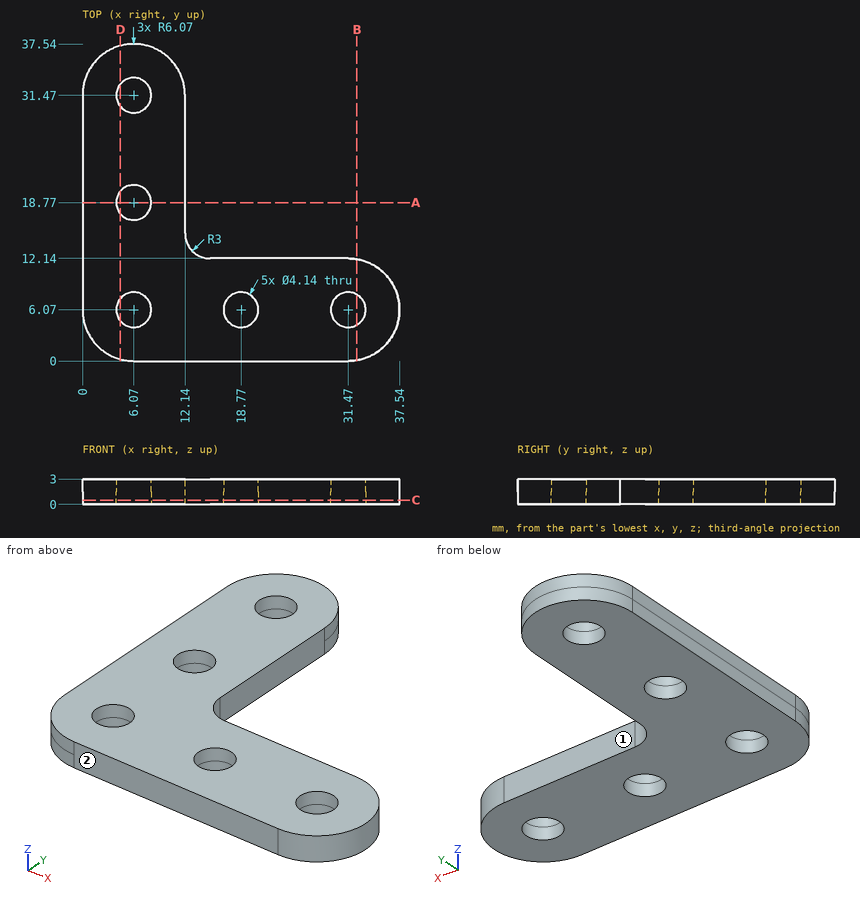
The figure shows three views and two pictorial views of one solid part (mm, origin at its lowest corner). Answer the questions. A direction names the side the tool comes from. Round coordinates to 2 decimals unless told otherwise and drop trailing zeros. Write each loop counter-clockwise with the first axis right and the second up, starting at its lowest first coordinate (ties: lowest second). Pieces come first, ordered by that corner, then holes. Notation, with made-up numbers: (-5.5, 21) -> (46.5, 21) arc R8 ccw to (46.5, 25) -> close; hole circle Ø6 at (65.25, -37). An arc over 180 degrees is marked (long way). Answer as a JSON object with one key per item and string values. Group by question number.
Q1. Section B-B (x = 32.5) is taken. Write down the section's boundary in (y, z).
Q2. Straight lines are drawn through the part: line 1 along Y through (x, z) = (31.47, 2.75); line 2 along X through (y, z) = (7.5, 0.7); line 3 along Y through (x, z) = (28.5, 1.6). For each, find the intervals that lie inside material, in ascending order.
Q3. Section D-D (x = 4.5) is taken. Write down the section's boundary in (y, z), plus the area to 3 significant figures.
Q4. Section A-A (y = 18.77) is taken. Write down the section's boundary in (x, z), plus the area to 3 significant figures.
Q5. Section C-C (z = 0.5) is taken. Write down the section's boundary in (x, y), plus the area to 3 significant figures.
Q6. Each of these flat-tipped pins is pushed along its axis until it touches: pin 1 Ø3.5 at (x, y) = (18.77, 6.07) entering from -Z; pin 2 Ø1 at (y, z) = (5, 2.5) entering from -X; pin 3 Ø0.9 at (y, z) = (25, 1.5) entering from +X. Where does it stop, or does it pass through?
Q7. Which of the six approach directions +Z, -Z, +X, -X, +Y, -Y give full straight-line access (tool end or side, diameter ignored) to the marked faces 1 and 2?
Check values:
{
 "1": {"outline": "(0.09, 0) -> (4.27, 0) -> (4.27, 3) -> (0.09, 3) -> close; (7.87, 0) -> (12.05, 0) -> (12.05, 3) -> (7.87, 3) -> close"},
 "2": {"line 1": "0 to 4, 8.14 to 12.14", "line 2": "0 to 4.57, 7.57 to 17.27, 20.27 to 29.97, 32.97 to 37.37", "line 3": "0 to 12.14"},
 "3": {"outline": "(0.21, 0) -> (4.72, 0) -> (4.72, 3) -> (0.21, 3) -> close; (7.42, 0) -> (17.42, 0) -> (17.42, 3) -> (7.42, 3) -> close; (20.12, 0) -> (30.12, 0) -> (30.12, 3) -> (20.12, 3) -> close; (32.82, 0) -> (37.33, 0) -> (37.33, 3) -> (32.82, 3) -> close", "area": "87.1 mm^2"},
 "4": {"outline": "(0, 0) -> (4, 0) -> (4, 3) -> (0, 3) -> close; (8.14, 0) -> (12.14, 0) -> (12.14, 3) -> (8.14, 3) -> close", "area": "24.0 mm^2"},
 "5": {"outline": "(0, 6.07) arc R6.07 ccw to (6.07, 0) -> (31.47, 0) arc R6.07 ccw to (31.47, 12.14) -> (15.14, 12.14) arc R3 cw to (12.14, 15.14) -> (12.14, 31.47) arc R6.07 ccw to (0, 31.47) -> close; hole circle Ø4.14 at (6.07, 6.07); hole circle Ø4.14 at (6.07, 18.77); hole circle Ø4.14 at (6.07, 31.47); hole circle Ø4.14 at (18.77, 6.07); hole circle Ø4.14 at (31.47, 6.07)", "area": "659 mm^2"},
 "6": {"pin 1": "through", "pin 2": "x = 0.03", "pin 3": "x = 12.14"},
 "7": {"face 1": "+Z, -Z, +X, +Y", "face 2": "+Z, -Z, +X, -X, -Y"}
}
